Can you work these out from the model? Positions are in its coordinate system, mm. A direction names the side the tool comes from. Give positions to 0.01 mm unless a question says otherwise; leave off trailing zeros. Order: outer loops, then holes, each group sorted by start corner. A loop starts at its lowest first (then second) coordinate and runs counter-clockwise, first axis right, second up. Notation, with made-up numbers: (36.25, -32) -> (44.25, -32) arc R19 ccw to (44.25, -25) -> close; hole circle Ø5 at (-1.5, 78). An arc over 180 degrees is marked (long way). Answer as CSV lines item,"result".
```python
from build123d import *

# Parameters (mm, degrees)
SKETCH_1_W          = 37.9
SKETCH_1_H          = 12.2
EXTRUDE_1_DEPTH     = 1.2
EXTRUDE_2_DEPTH     = 1.8
FILLET_1_R          = 0.9
SKETCH_4_R          = 0.7
CUT_EXTRUDE_1_DEPTH = 22.034554904
SKETCH_5_W          = 2.8
SKETCH_5_H          = 10.1
SKETCH_5_H_2        = 8
SKETCH_5_W_2        = 4
SKETCH_5_H_3        = 7.4
EXTRUDE_3_DEPTH     = 0.8


with BuildPart() as part:
    # Эскиз1 → Бобышка-Вытянуть1 (new body)
    with BuildSketch(Plane(origin=(0, 0, 0), x_dir=(1, 0, 0), z_dir=(0, 1, 0))):
        Rectangle(SKETCH_1_W, SKETCH_1_H)
    extrude(amount=EXTRUDE_1_DEPTH)

    # Эскиз2 → Бобышка-Вытянуть2 (add)
    with BuildSketch(Plane(origin=(0, 1.2, 0), x_dir=(1, 0, 0), z_dir=(0, 1, 0))):
        Polygon((-12.95, 5.85), (17.05, 5.85), (17.05, 1.15), (20.05, 1.15), (20.05, -5.85), (17.05, -5.85), (-12.95, -5.85), align=None)
    extrude(amount=EXTRUDE_2_DEPTH)

    # Скругление1
    fillet_1_edges = [part.edges().sort_by_distance(p)[0] for p in [
        (20.05, 1.2, 2.35),
        (20.05, 3, 2.35),
    ]]
    fillet(fillet_1_edges, radius=FILLET_1_R - 0.0001)  # a hair under: the kernel refuses the full size

    # Эскиз4 → Вырез-Вытянуть1 (cut, through all)
    with BuildSketch(Plane(origin=(0, 1.2, 0), x_dir=(1, 0, 0), z_dir=(0, 1, 0))):
        with Locations(Location((-17.55, 3.81, 0), (0, 0, 270))):
            Circle(SKETCH_4_R)
        with Locations(Location((-17.55, 1.27, 0), (0, 0, 270))):
            Circle(SKETCH_4_R)
        with Locations(Location((-17.55, -1.27, 0), (0, 0, 270))):
            Circle(SKETCH_4_R)
        with Locations(Location((-17.55, -3.81, 0), (0, 0, 270))):
            Circle(SKETCH_4_R)
    extrude(amount=-CUT_EXTRUDE_1_DEPTH, mode=Mode.SUBTRACT)

    # Эскиз5 → Бобышка-Вытянуть3 (add)
    with BuildSketch(Plane.XZ):
        with Locations((5.05, 0.35)):
            Rectangle(SKETCH_5_W, SKETCH_5_H)
        with Locations((-2.05, 0.7)):
            Rectangle(SKETCH_5_W, SKETCH_5_H_2)
        with Locations((-9.55, 0.6)):
            Rectangle(SKETCH_5_W_2, SKETCH_5_H_3)
    extrude(amount=EXTRUDE_3_DEPTH)


solid = part.part
```
Item 1: For pin 1 (2 mm diameter, centred on y = 0, z = -0.5, fed in from +X); pin 2 (1.4 mm diameter, centred on y = 2, z = -3, fed in from +X); pin 3 (0.6 mm diameter, centred on x = -1.5, y = -0.5, fed in from -Z); pin 4 (1.5 mm diameter, centred on y = -0.5, z = 0, fed in from -X), each with a flat end and sliding along its axis, tell me the tip position at first contact or that it passes through.
Numbers:
pin 1,"stops at x = 18.95"
pin 2,"stops at x = 17.05"
pin 3,"stops at z = -3.3"
pin 4,"stops at x = -18.95"
Item 2: Imagine slicing it at B-B, the plane x = -17.55. Please give me the cut outline in (y, z).
Numbers:
outline,"(0, -6.1) -> (1.2, -6.1) -> (1.2, -4.51) -> (0, -4.51) -> close; (0, -3.11) -> (1.2, -3.11) -> (1.2, -1.97) -> (0, -1.97) -> close; (0, -0.57) -> (1.2, -0.57) -> (1.2, 0.57) -> (0, 0.57) -> close; (0, 1.97) -> (1.2, 1.97) -> (1.2, 3.11) -> (0, 3.11) -> close; (0, 4.51) -> (1.2, 4.51) -> (1.2, 6.1) -> (0, 6.1) -> close"
Item 3: Please list where these lines run through material, in increasing order: line 1 along X through (y, z) = (-0.5, 1.75); line 2 along X through (y, z) = (0.5, 3.81); line 3 along Y through (x, z) = (14, -4).
Numbers:
line 1,"x = -11.55 to -7.55, -3.45 to -0.65, 3.65 to 6.45"
line 2,"x = -18.95 to -18.25, -16.85 to 18.95"
line 3,"y = 0 to 3"
Item 4: Imagine slicing it at C-C, the plane z = -3.81. Please give me the cut outline in (x, y).
Numbers:
outline,"(-18.95, 0) -> (-18.25, 0) -> (-18.25, 1.2) -> (-18.95, 1.2) -> close; (-16.85, 0) -> (3.65, 0) -> (3.65, -0.8) -> (6.45, -0.8) -> (6.45, 0) -> (18.95, 0) -> (18.95, 1.2) -> (17.05, 1.2) -> (17.05, 3) -> (-12.95, 3) -> (-12.95, 1.2) -> (-16.85, 1.2) -> close"
Item 5: For faces 4 (the flat face through (2, 2, -5.85)), 5 (the flat face through (19, 2, -1.15)), 6 (the flat face through (3, 2, 5.85)), 7 (the flat face through (-18.95, 1, 0)), 8 (the flat face through (-12.95, 2, 0)), which set-ups out of +Z, -Z, +X, -X, +Y, -Y let a thin tool reach every point of the face, with its end or its side?
Numbers:
face 4,"-Z, +X, -X, +Y"
face 5,"-Z, +X, +Y"
face 6,"+Z, +X, -X, +Y"
face 7,"+Z, -Z, -X, +Y, -Y"
face 8,"+Z, -Z, -X, +Y"
Item 6: We'd pull the mould along X, two halves only. Please class faces 1 (the flat face through (-2, -0.8, 1)), 2 (the cylindrical face through (-18.233, 0.608, -3.962)), 3 (the flat face through (18.95, 1, 0)): released by +X, released by -X, zero draft, split by the parting line, or undercut.
Numbers:
face 1,"zero draft"
face 2,"undercut"
face 3,"released by +X"
Item 7: Imagine slicing it at D-D, the plane x = 0. Please give me the cut outline in (y, z).
Numbers:
outline,"(0, -6.1) -> (1.2, -6.1) -> (1.2, -5.85) -> (3, -5.85) -> (3, 5.85) -> (1.2, 5.85) -> (1.2, 6.1) -> (0, 6.1) -> close"
